The drawing under review shows one solid part. Ordinate dimensions are in mm from its lowest x, y, z. A direction names the side the tool comes from. Coordinates: 2 decimals unless noted, no trailing zeros. Write each loop counter-clockwise with the first axis right and the second up, starting at its lowest first coordinate (ties: lowest second). Pieces come first, ordered by that corner, then holes. Notation, with made-up numbers: (29.25, -22) - (66.25, -22) arc R35 ccw to (66.25, 14) - close; hole circle Ø1 at (-13.75, 37.5). An arc over 180 degrees is marked (long way). Put each result on its own line as item: value. Start each with the question number.
Item 1: Consider section A-A on y = 22.5. Give the boundary of the cut face in (x, z), then the cut area to 3 significant figures.
Item 2: Mouldability with a two-part tool opening along X and no side actions: class the marked faces 1, 2, 3 and 4 as pulls with the +X half, pulls with the -X half, needs draft (parallel to the pull), parting line crosses it, or undercut.
Item 3: For pin 1 (12.5 mm diameter, centred on y = 42.5, z = 33, fed in from +X); pin 2 (1 mm diameter, centred on x = 57, y = 48, fed in from +Z); pin 3 (6.5 mm diameter, centred on x = 20.5, z = 36, fed in from -Y), all flat-tipped, find the tip position at first contact; note any pin that passes through.
Item 4: To check wall thickness, follow L1, parallel to X at y = 33, z = 34.5; L2, parallel to X at y = 6, z = 46; L3, parallel to Y at x = 13.5, z = 28. State the ranges of each line that lie inside material, in increasing order. Write a range as [from, to].
Item 5: Machinability: for the marked faces 5, 6 and 7, which of the approach directions +Z, -Z, +X, -X, +Y, -Y give a long, thin tool a straight path to every point of the face, cutting with its end or side? Answer none if there is none.
Item 6: Consider section C-C on z = 46.5. Give the boundary of the cut face in (x, y).
Item 7: Consider section B-B on x = 47. Give the boundary of the cut face in (y, z).
Item 8: Consider section D-D on y = 47. Give the boundary of the cut face in (x, z).
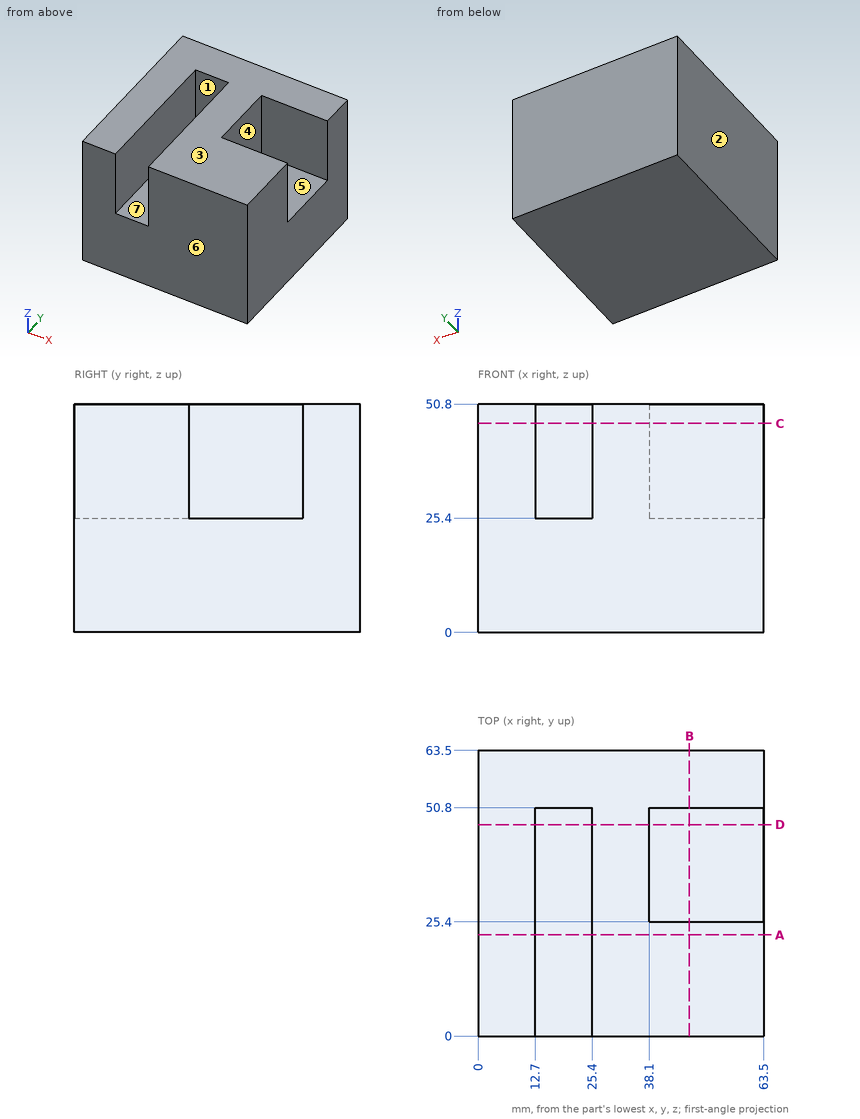
Report:
1. outline: (0, 0) - (63.5, 0) - (63.5, 50.8) - (25.4, 50.8) - (25.4, 25.4) - (12.7, 25.4) - (12.7, 50.8) - (0, 50.8) - close
1. area: 2,900 mm²
2. face 1: undercut
2. face 2: pulls with the -X half
2. face 3: needs draft
2. face 4: pulls with the +X half
3. pin 1: x = 38.1
3. pin 2: z = 25.4
3. pin 3: y = 50.8
4. L1: [0, 12.7], [25.4, 38.1]
4. L2: [0, 12.7], [25.4, 63.5]
4. L3: [50.8, 63.5]
5. face 5: +Z, +X
5. face 6: +Z, -Z, +X, -X, -Y
5. face 7: +Z, -Y
6. outline: (0, 0) - (12.7, 0) - (12.7, 50.8) - (25.4, 50.8) - (25.4, 0) - (63.5, 0) - (63.5, 25.4) - (38.1, 25.4) - (38.1, 50.8) - (63.5, 50.8) - (63.5, 63.5) - (0, 63.5) - close
7. outline: (0, 0) - (63.5, 0) - (63.5, 50.8) - (50.8, 50.8) - (50.8, 25.4) - (25.4, 25.4) - (25.4, 50.8) - (0, 50.8) - close
8. outline: (0, 0) - (63.5, 0) - (63.5, 25.4) - (38.1, 25.4) - (38.1, 50.8) - (25.4, 50.8) - (25.4, 25.4) - (12.7, 25.4) - (12.7, 50.8) - (0, 50.8) - close
